from build123d import *

# Parameters (mm, degrees)
SKETCH_1_R      = 1.6
SKETCH_1_R_2    = 16
SKETCH_1_R_3    = 2.1
EXTRUDE_1_DEPTH = 4


with BuildPart() as part:
    # 草图1 → 凸台-拉伸1 (new body)
    with BuildSketch(Plane(origin=(0, 0, 0), x_dir=(1, 0, 0), z_dir=(0, 1, 0))):
        with BuildLine():
            Line((0, 0), (42, 0))
            Line((42, 0), (42, -57))
            ThreePointArc((42, -57), (40.535533906, -60.535533906), (37, -62))
            Line((37, -62), (5, -62))
            ThreePointArc((5, -62), (1.464466094, -60.535533906), (0, -57))
            Line((0, -57), (0, 0))
        make_face()
        with Locations(Location((5.5, -25.5, 0), (0, 0, 270))):
            Circle(SKETCH_1_R, mode=Mode.SUBTRACT)
        with Locations(Location((36.5, -25.5, 0), (0, 0, 270))):
            Circle(SKETCH_1_R, mode=Mode.SUBTRACT)
        with Locations(Location((36.5, -56.5, 0), (0, 0, 270))):
            Circle(SKETCH_1_R, mode=Mode.SUBTRACT)
        with Locations(Location((5.5, -56.5, 0), (0, 0, 270))):
            Circle(SKETCH_1_R, mode=Mode.SUBTRACT)
        with Locations(Location((21, -41, 0), (0, 0, 270))):
            Circle(SKETCH_1_R_2, mode=Mode.SUBTRACT)
        with Locations(Location((21, -10, 0), (0, 0, 270))):
            Circle(SKETCH_1_R_3, mode=Mode.SUBTRACT)
        with Locations(Location((36, -10, 0), (0, 0, 270))):
            Circle(SKETCH_1_R_3, mode=Mode.SUBTRACT)
        with Locations(Location((6, -10, 0), (0, 0, 270))):
            Circle(SKETCH_1_R_3, mode=Mode.SUBTRACT)
    extrude(amount=EXTRUDE_1_DEPTH)


solid = part.part
Model file for the job. Use its own axes, mm. Give positions to 0.01 mm unless a question says otherwise; leave off trailing zeros. Order: outer loops, then holes, each group sorted by start corner. A loop starts at its lowest first (then second) coordinate and runs counter-clockwise, first axis right, second up. Notation, with made-up numbers: M -37.75,17 L 17.25,17 A30 cw 17.25,43 Z; hole C 26,4.25 d6. An arc over 180 degrees is marked long. Put each result on its own line as item: value. Start each with the question number.
(1) Drill centre lines: L1, parallel to X at y = 3.2, z = 10; L2, parallel to X at y = 3.1, z = 41; L3, parallel to Z at x = 35.5, y = 0.55. Where is each one in solid material? Low to high. Write a range as [from, to].
(2) Band-saw the part on B-B on z = 10. Give the cut face in (x, y), then the cut area to 3 significant figures.
(3) Pull direction Z, two halves, no side cores. Call faces 1 (the face through (42, 2, 28)), 2 (the face through (4.89, 1.97, 57.98)), 3 (the face through (41, 2, 60)): released by +Z, released by -Z, zero draft, split by the parting line, or undercut.
(4) Band-saw the part on D-D on y = 1.05. Count the separate pieces of the cut face and the enclosed holes in it, then the cut area to 3 significant figures.
(5) Band-saw the part on C-C on z = 41. Give the cut face in (x, y).
(6) Band-saw the part on A-A on x = 21. Give the cut face in (y, z).
Results below:
1. L1: x = [0, 3.9], [8.1, 18.9], [23.1, 33.9], [38.1, 42]
1. L2: x = [0, 5], [37, 42]
1. L3: z = [0, 7.96], [12.04, 24.25], [26.75, 34.24], [47.76, 55.25], [57.75, 62]
2. outline: M 0,0 L 3.9,0 L 3.9,4 L 0,4 Z; M 8.1,0 L 18.9,0 L 18.9,4 L 8.1,4 Z; M 23.1,0 L 33.9,0 L 33.9,4 L 23.1,4 Z; M 38.1,0 L 42,0 L 42,4 L 38.1,4 Z
2. area: 118 mm2
3. face 1: zero draft
3. face 2: undercut
3. face 3: released by +Z
4. separate pieces: 1
4. enclosed holes: 8
4. area: 1,720 mm2
5. outline: M 0,0 L 5,0 L 5,4 L 0,4 Z; M 37,0 L 42,0 L 42,4 L 37,4 Z
6. outline: M 0,0 L 4,0 L 4,7.9 L 0,7.9 Z; M 0,12.1 L 4,12.1 L 4,25 L 0,25 Z; M 0,57 L 4,57 L 4,62 L 0,62 Z
